```python
from build123d import *

# Parameters (mm, degrees)
CHAMFER1_SIZE      = 0.5
CUT_EXTRUDE1_DEPTH = 2.4


with BuildPart() as part:
    # Sketch1 → Revolve1 (revolve)
    with BuildSketch(Plane.XY, mode=Mode.PRIVATE) as revolve1_sk:
        with BuildLine():
            Line((0, 0), (0, 4.5))
            ThreePointArc((0, 4.5), (-0.146446609, 4.853553391), (-0.5, 5))
            Line((-0.5, 5), (-4.5, 5))
            Line((-4.5, 5), (-4.5, 2.5))
            Line((-4.5, 2.5), (-14.5, 2.5))
            Line((-14.5, 2.5), (-14.5, 2))
            Line((-14.5, 2), (-22.5, 2))
            Line((-22.5, 2), (-22.5, 0))
            Line((-22.5, 0), (0, 0))
        make_face()
    revolve(revolve1_sk.sketch.rotate(Axis((0, 0, 0), (1, 0, 0)), 90), axis=Axis((0, 0, 0), (1, 0, 0)))

    # Chamfer1
    chamfer1_edges = [part.edges().sort_by_distance(p)[0] for p in [
        (-22.5, 0, -2),
    ]]
    chamfer(chamfer1_edges, length=CHAMFER1_SIZE)

    # Sketch2 → Cut-Extrude1 (cut)
    with BuildSketch(Plane(origin=(0, 0, 0), x_dir=(0, 0, -1), z_dir=(1, 0, 0))):
        Polygon((1.732050808, 0), (0.866025404, 1.5), (-0.866025404, 1.5), (-1.732050808, 0), (-0.866025404, -1.5), (0.866025404, -1.5), align=None)
    extrude(amount=-CUT_EXTRUDE1_DEPTH, mode=Mode.SUBTRACT)


solid = part.part
```
Design review of the part built by this model. Coordinates are the model's own, in mm. A direction names the side the tool comes from. Round coordinates to 2 decimals unless told otherwise and drop trailing zeros. Order: outer loops, then holes, each group sorted by start corner. A loop starts at its lowest first (then second) coordinate and runs counter-clockwise, first axis right, second up. Notation, with made-up numbers: (24.5, -18) - (63.5, -18) arc R29 ccw to (63.5, 13) - close; hole circle Ø10 at (86.25, 13.25). An arc over 180 degrees is marked (long way). Return JSON: item names as keys, results as strings.
Q1. Machinability: for faces 1 (the cylindrical face through (-3, 0, -5)), 2 (the flat face through (-1, 1.5, 0)), 3 (the cylindrical face through (-9.6, -0.1, -2.5)), which of the approach directions +Z, -Z, +X, -X, +Y, -Y give a long, thin tool a straight path to every point of the face, cutting with its end or side? Answer none if there is none.
Computed values:
{"face 1": "+X, -X", "face 2": "+X", "face 3": "-X"}
Q2. Consider section B-B on x = -18. Write out the cut boundary in (y, z).
Computed values:
{"outline": "circle Ø4 at (0, 0)"}
Q3. For pin 1 Ø1 at (x, z) = (-9.5, -0.5) entering from -Y; pin 2 Ø3.5 at (y, z) = (0, 0) entering from +X; pin 3 Ø5 at (x, y) = (-18.5, 2.5) entering from -Z, all flat-tipped, find the tip position at first contact; note any pin that passes through.
Computed values:
{"pin 1": "stops at y = -2.5", "pin 2": "stops at x = 0", "pin 3": "stops at z = -2"}
Q4. Wall thickness on L1, parallel to X at y = -1, z = 2; L2, parallel to X at y = 0.5, z = -3.75; L3, parallel to Y at x = -9, z = 1.5: over which ranges is each line inside the solid? List them lowest first. Write a range as [from, to].
Computed values:
{"L1": "x = [-14.5, 0]", "L2": "x = [-4.5, 0]", "L3": "y = [-2, 2]"}
Q5. Consider section C-C on x = -8. Write out the cut boundary in (y, z).
Computed values:
{"outline": "circle Ø5 at (0, 0)"}
Q6. Consider section A-A on z = 0. Write out the cut boundary in (x, y).
Computed values:
{"outline": "(-22.5, -1.5) - (-22, -2) - (-14.5, -2) - (-14.5, -2.5) - (-4.5, -2.5) - (-4.5, -5) - (-0.5, -5) arc R0.5 ccw to (0, -4.5) - (0, -1.5) - (-2.4, -1.5) - (-2.4, 1.5) - (0, 1.5) - (0, 4.5) arc R0.5 ccw to (-0.5, 5) - (-4.5, 5) - (-4.5, 2.5) - (-14.5, 2.5) - (-14.5, 2) - (-22, 2) - (-22.5, 1.5) - close"}
Q7. The part is to be moulded in two halves that separate along Z. For faces 4 (the cylindrical face through (-18, 2, 0)), 5 (the flat face through (-4.5, 2, 2)), 6 (the flat face through (-1.183, 0.74, -1.305)), say which applies: pulls with the +Z half, pulls with the -Z half, needs draft (parallel to the pull), parting line crosses it, or undercut.
Computed values:
{"face 4": "parting line crosses it", "face 5": "needs draft", "face 6": "undercut"}
